```python
from build123d import *

# Parameters (mm, degrees)
F0_W     = 41.957522
F0_H     = 100
F1_DEPTH = 3
F3_D     = 5
F6_DEPTH = 25
F7_R     = 10


with BuildPart() as f1:
    # F0 (on Top) → F1 (new body)
    with BuildSketch(Plane.XY):
        with Locations((20.978761, 50)):
            Rectangle(F0_W, F0_H)
    extrude(amount=F1_DEPTH)

    # F3 (through all)
    with Locations(Plane.XY.offset(3)):
        with Locations((11.957522, 50), (11.957522, 25)):
            Hole(F3_D / 2)

    # F5 (on face) → F6 (cut)
    with BuildSketch(Plane.XY.offset(3)):
        with BuildLine():
            ThreePointArc((29.457522, 20), (31.957522, 17.5), (34.457522, 20))
            Line((34.457522, 20), (34.457522, 60))
            ThreePointArc((34.457522, 60), (31.957522, 62.5), (29.457522, 60))
            Line((29.457522, 60), (29.457522, 20))
        make_face()
    extrude(amount=-F6_DEPTH, mode=Mode.SUBTRACT)

    # F7
    f7_edges = [f1.edges().sort_by_distance(p)[0] for p in [
        (41.957522, 0, 1.5),
        (41.957522, 100, 1.5),
    ]]
    fillet(f7_edges, radius=F7_R)

    # F8: F1 across plane


with BuildPart() as f1_1:
    add(f1.part)
    add(f1.part.mirror(Plane.YZ))


solid = f1_1.part
```
Input: part model. Units: mm. Frame: model coordinates. A direction names the side the tool comes from. Round coordinates to 2 decimals unless told otherwise and drop trailing zeros. Loops run counter-clockwise (first coordinate to the right, second up) from the corner with the lowest first, then second, coordinate; pieces in that order, holes last. Notation, with made-up numbers: (-23.75, 60) -> (13.25, 60) arc R15 cw to (13.25, 73) -> close; hole circle Ø1 at (5.25, 54.25). An arc over 180 degrees is marked (long way). Write each question's results on one line, items separated by ' | '.
1. Set-up query: faces 1 (the face through (31.9, 17.5, 1.5)), 2 (the face through (1, 51, 0)). Return all of +Z, -Z, +X, -X, +Y, -Y with unobstructed straight access to the full face (end or side cutting, diameter ignored); none if empty.
Geometry results:
face 1: +Z, -Z | face 2: -Z, +X, -X, +Y, -Y
2. First-contact query: P1, Ø4, axis at x = 32.5, y = 86.5, coming from the -Z side; P2, Ø4, axis at x = -11.96, y = 25, coming from the -Z side. Flat tips, straight axial feed; report the tip coordinate or a pass-through.
Geometry results:
P1: z = 0 | P2: through
3. Ray query, line 1 (X direction, y = 40.5, z = 0.65); line 2 (Y direction, x = -10.5, z = 1.3); line 3 (Y direction, x = 11.5, z = 1.5). Return the intervals inside material, ascending. Write a range as from..to.
Geometry results:
line 1: -41.96..-34.46, -29.46..29.46, 34.46..41.96 | line 2: 0..22.97, 27.03..47.97, 52.03..100 | line 3: 0..22.54, 27.46..47.54, 52.46..100
4. Section D-D (x = 12.5). Return loops of the section in (y, z), and give its area (3 significant figures).
Geometry results:
outline: (0, 0) -> (22.56, 0) -> (22.56, 3) -> (0, 3) -> close; (27.44, 0) -> (47.56, 0) -> (47.56, 3) -> (27.44, 3) -> close; (52.44, 0) -> (100, 0) -> (100, 3) -> (52.44, 3) -> close | area: 271 mm2
5. Mould query, pull axis Y, two halves, no side actions, for faces 3 (the face through (39, 97.1, 1.5)), 4 (the face through (-39, 2.9, 1.5)), 5 (the face through (-32, 62.5, 1.5)), 6 (the face through (32, 62.5, 1.5)). Classes: +Y half, -Y half, draft (parallel to the pull), parting line (faces both ways), or undercut.
Geometry results:
face 3: +Y half | face 4: -Y half | face 5: undercut | face 6: undercut
6. Section B-B (y = 36). Return loops of the section in (x, z).
Geometry results:
outline: (-41.96, 0) -> (-34.46, 0) -> (-34.46, 3) -> (-41.96, 3) -> close; (-29.46, 0) -> (29.46, 0) -> (29.46, 3) -> (-29.46, 3) -> close; (34.46, 0) -> (41.96, 0) -> (41.96, 3) -> (34.46, 3) -> close
7. Section A-A (y = 50). Return loops of the section in (x, z).
Geometry results:
outline: (-41.96, 0) -> (-34.46, 0) -> (-34.46, 3) -> (-41.96, 3) -> close; (-29.46, 0) -> (-14.46, 0) -> (-14.46, 3) -> (-29.46, 3) -> close; (-9.46, 0) -> (9.46, 0) -> (9.46, 3) -> (-9.46, 3) -> close; (14.46, 0) -> (29.46, 0) -> (29.46, 3) -> (14.46, 3) -> close; (34.46, 0) -> (41.96, 0) -> (41.96, 3) -> (34.46, 3) -> close
8. Section C-C (z = 1.6). Return loops of the section in (x, y).
Geometry results:
outline: (-41.96, 10) arc R10 ccw to (-31.96, 0) -> (31.96, 0) arc R10 ccw to (41.96, 10) -> (41.96, 90) arc R10 ccw to (31.96, 100) -> (-31.96, 100) arc R10 ccw to (-41.96, 90) -> close; hole (-34.46, 20) arc R2.5 ccw to (-29.46, 20) -> (-29.46, 60) arc R2.5 ccw to (-34.46, 60) -> close; hole circle Ø5 at (-11.96, 25); hole circle Ø5 at (-11.96, 50); hole circle Ø5 at (11.96, 25); hole circle Ø5 at (11.96, 50); hole (29.46, 20) arc R2.5 ccw to (34.46, 20) -> (34.46, 60) arc R2.5 ccw to (29.46, 60) -> close
